from build123d import *

# Parameters (mm, degrees)
F0_W     = 88.9
F0_H     = 38.1
F1_DEPTH = 1676.4
F3_DEPTH = 84.074
F4_R     = 5.08


with BuildPart() as f1:
    # F0 (on Front) → F1 (new body)
    with BuildSketch(Plane.XZ):
        with Locations((44.45, 19.05)):
            Rectangle(F0_W, F0_H)
    extrude(amount=F1_DEPTH)

    # F2 (on face) → F3 (cut)
    with BuildSketch(Plane.XY.offset(38.1)):
        Polygon((88.9, -1640.120582), (0, -1676.4), (88.9, -1676.4), align=None)
    extrude(amount=-F3_DEPTH, mode=Mode.SUBTRACT)

    # F4
    f4_edges = [f1.edges().sort_by_distance(p)[0] for p in [
        (0, -838.2, 38.1),
        (88.9, -820.060291, 38.1),
        (0, -838.2, 0),
        (88.9, -820.060291, 0),
    ]]
    fillet(f4_edges, radius=F4_R)


solid = f1.part
For this review, take the finished solid that the model builds, in its own axes (mm). Give positions to 0.01 mm unless a question says otherwise; leave off trailing zeros. Loops run counter-clockwise (first coordinate to the right, second up) from the corner with the lowest first, then second, coordinate; pieces in that order, holes last.
Item 1: Take a section at A-A, the plane x = 67. State the section outline as (y, z) points.
Item 2: Insertion check: pin 1 (10 mm diameter, centred on x = 79, z = 31, fed in from +Y); pin 2 (6 mm diameter, centred on x = 47, z = 32.5, fed in from -Y). Each pin has a flat end and moves straight along its axis. Give the tip position at first contact, or say it passes through.
Item 3: For line 1 along Y through (x, z) = (12, 28.5); line 2 along Z through (x, y) = (4.5, -420.5); line 3 along Y through (x, z) = (23.5, 17), list the stretches that pass through material, from the lowest coordinate up.
Calculated:
1. outline: (-1649.06, 0) - (0, 0) - (0, 38.1) - (-1649.06, 38.1) - close
2. pin 1: stops at y = 0
2. pin 2: stops at y = -1658.44
3. line 1: y = -1671.5 to 0
3. line 2: z = 0.03 to 38.07
3. line 3: y = -1666.81 to 0
